Job drawing, mm, ordinate dimensions from the low corner. One solid piece. A direction names the side the tool comes from. Give positions to 0.01 mm unless a question says otherwise; leave off trailing zeros. Order: outer loops, then holes, each group sorted by start corner. A loop starts at its lowest first (then second) coordinate and runs counter-clockwise, first axis right, second up. Notation, with made-up numbers: (88, 4) - (143, 4) arc R34 ccw to (143, 37) - close; hole circle Ø7 at (-20.5, 3.5). An arc over 180 degrees is marked (long way). One line per item, written item: value.
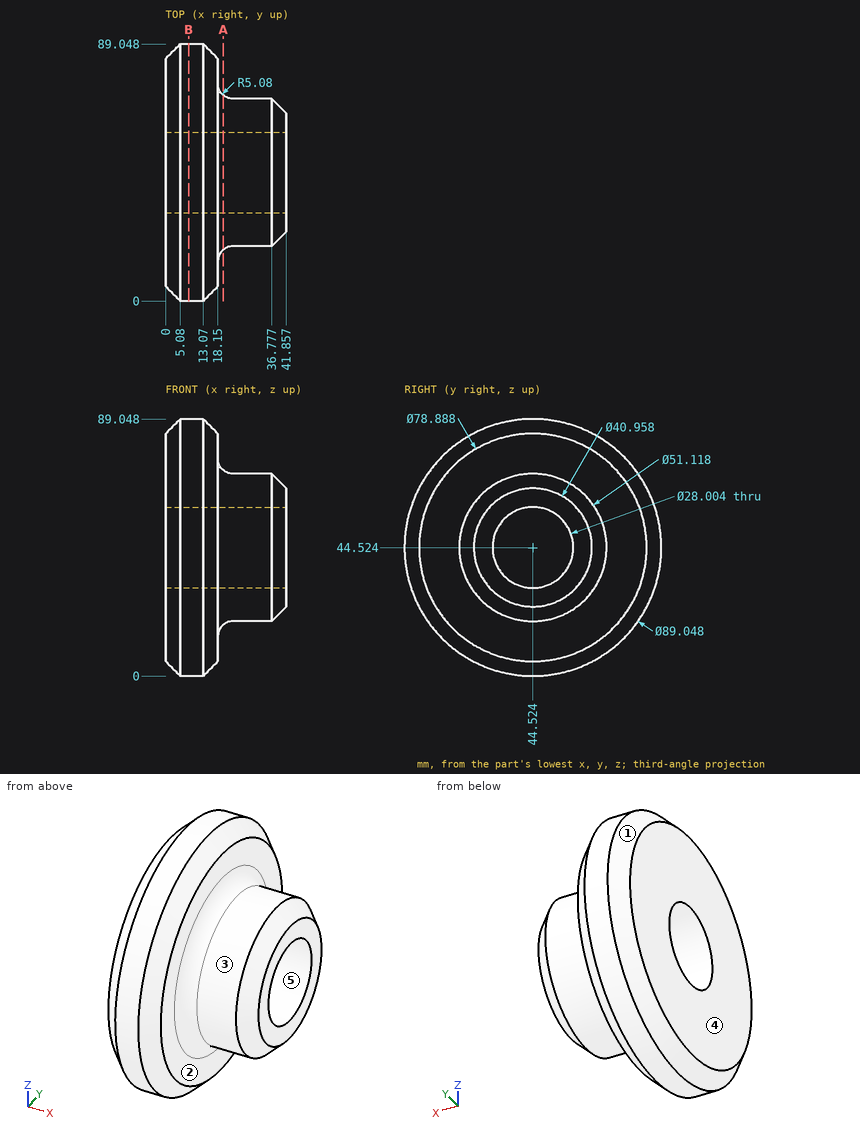
1) Which spindle directions (+Z, -Z, +X, -X, +Y, -Y) get a long thin tool onto all of the face, cutting with end or side? Do the marked faces 1 and 2. Say none if no direction does.
Answer:
face 1: -X
face 2: +X
2) Drop flat-ended pins along their axis: P1, Ø6, axis at x = 16.5, z = 61.5, coming from the -Y side; P2, Ø10, axis at x = 6.5, y = 65, coming from the -Z side; P3, Ø8, axis at x = 8.5, z = 63, coming from the +Y side. Give the stop position or say it passes through.
Answer:
P1: stops at y = 3.61
P2: stops at z = 2.78
P3: stops at y = 86.63
3) Wall check: line 1 along Y through (x, z) = (20.5, 36) (1 decimal); line 2 along X through (y, z) = (52.5, 8); line 3 along Z through (x, y) = (14, 63). Give the ranges that are in metal, low to high. Write a range as [from, to].
Answer:
line 1: y = [19.6, 33.4], [55.6, 69.5]
line 2: x = [0, 18.15]
line 3: z = [5.04, 84.01]
4) Two-plate mould, pull along Z, no slides. Class the marked faces 3, 4 and 5: pulls with the +Z half, pulls with the -Z half, needs draft (parallel to the pull), parting line crosses it, or undercut.
Answer:
face 3: parting line crosses it
face 4: needs draft
face 5: undercut
5) Slice it at B-B on x = 8. Write the cut outline in (y, z) (1 decimal).
Answer:
outline: circle Ø89 at (44.5, 44.5); hole circle Ø28 at (44.5, 44.5)
6) Slice it at A-A on x = 20. Write the cut outline in (y, z) (1 decimal).
Answer:
outline: circle Ø53.4 at (44.5, 44.5); hole circle Ø28 at (44.5, 44.5)
